Source: three-view drawing plus pictorial views. Frame: mm from the lowest corner of the part. Give positions to 0.01 mm unless a question says otherwise; leave off trailing zeros. Put each result on its own line as item: value.
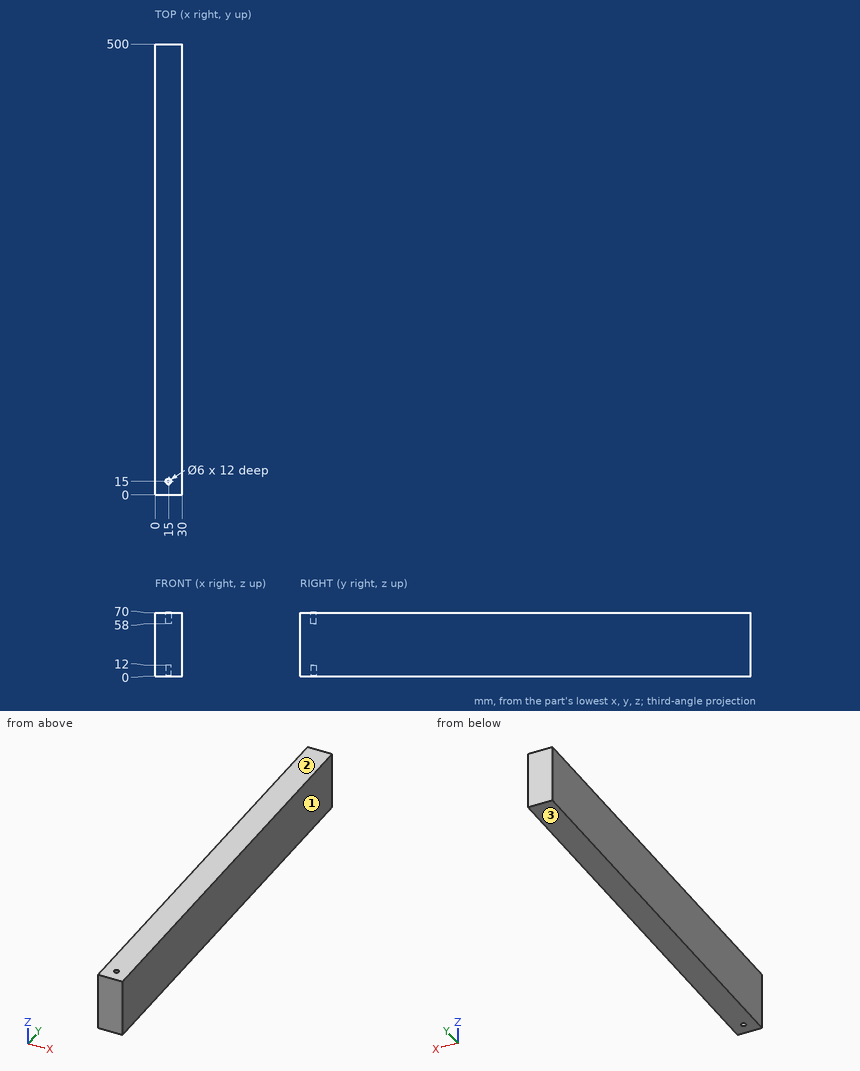
(1) First-contact query: P1, Ø10, axis at y = 330.5, z = 40.5, coming from the -X side; P2, Ø3, axis at x = 15.5, y = 15.5, coming from the -Z side; P3, Ø5, axis at x = 15, y = 15, coming from the +Z side. Flat tips, straight axial feed; report the tip coordinate or a pass-through.
Calculated:
P1: stops at x = 0
P2: stops at z = 12
P3: stops at z = 58
(2) Line query: probe 1 along Y at (x, z) = (15, 6.5); probe 2 along X at (y, z) = (15, 5); probe 3 along Y at (x, z) = (12.25, 60.5). Output: solid intervals per line, ascending. Write a range as from..to.
Calculated:
probe 1: y = 0..12, 18..500
probe 2: x = 0..12, 18..30
probe 3: y = 0..13.8, 16.2..500
(3) Draft query along Z for the marked faces 1, 2 and 3. Return one class per face: released by +Z, released by -Z, zero draft, split by the parting line, or undercut.
Calculated:
face 1: zero draft
face 2: released by +Z
face 3: released by -Z
